Autodesk Inventor part; units mm, degrees
ref_plane "YZ Plane" through (0, 0, 0) normal (1, 0, 0) x (0, 1, 0)
ref_plane "XZ Plane" through (0, 0, 0) normal (0, 1, 0) x (-1, 0, 0)
ref_plane "XY Plane" through (0, 0, 0) normal (0, 0, 1) x (1, 0, 0)
sketch "Sketch1" plane through (0, 0, 0) normal (0, 0, 1) x (1, 0, 0)
  line L0 (0, 0) -> (76, 0)
  line L1 (76, 0) -> (76, -8)
  line L2 (76, -8) -> (0, -8)
  line L3 (0, -8) -> (0, 0)
  dimension "d0" = 76
  dimension "d1" = 8
extrude "Extrusion1" add sketch "Sketch1" along normal blind 3
sketch "Sketch2" plane through (0, 0, 3) normal (0, 0, 1) x (1, 0, 0)
  line L0 (0, 0) -> (0, -8)
  circle A0 centre (0, -4) radius 1.9
  line L1 (76, -8) -> (76, 0)
  circle A1 centre (76, -4) radius 1.9
  dimension "d4" = 3.8
  dimension "d5" = 3.8
extrude "Extrusion2" add sketch "Sketch2" along normal blind 6
sketch "Sketch3" plane through (0, 0, 0) normal (0, 0, -1) x (-1, 0, 0)
  line L0 (0, -8) -> (-76, -8)
  line L1 (0, -8) -> (2.5, -8)
  line L2 (2.5, -8) -> (2.5, 0)
  line L3 (2.5, 0) -> (0, 0)
  line L4 (0, 0) -> (0, -8)
  line L5 (-76, -8) -> (-78.5, -8)
  line L6 (-78.5, -8) -> (-78.5, 0)
  line L7 (-78.5, 0) -> (-76, 0)
  line L8 (-76, 0) -> (-76, -8)
  dimension "d8" = 2.5
  dimension "d9" = 2.5
extrude "Extrusion3" add sketch "Sketch3" against normal blind 3
properties part number "SteeringWheel"
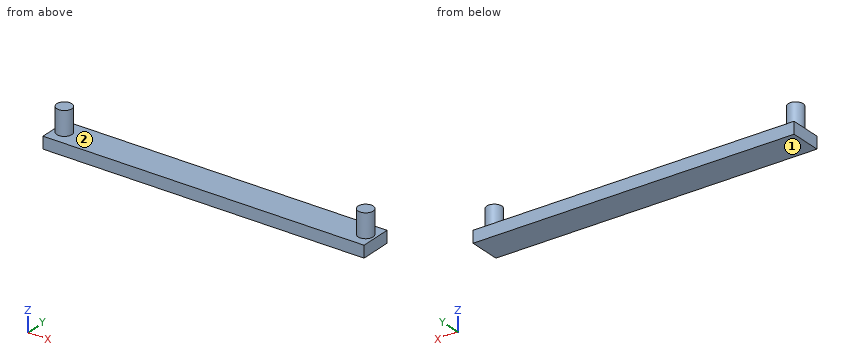
Source: CAD feature listing. Evaluate the final solid. Frame: model axes, mm. Face numbers are marked on the shaded views. Coordinates: 2 decimals unless noted, no trailing zeros. Write each loop counter-clockwise with the first axis right and the second up, starting at its lowest first coordinate (ties: lowest second). Pieces come first, ordered by that corner, then holes. Notation, with made-up numbers: M 60,-24.5 L 107,-24.5 A19 ccw 107,-6.5 Z; hole C 69,67 d6. An arc over 180 degrees is marked long. Use a Markdown table: item, result.
1) Section D-D, the plane x = 25.5. Output: boundary loops of the cut face in (y, z).
Conclusion:
| item | result |
|---|---|
| outline | M -8,0 L 0,0 L 0,3 L -8,3 Z |
2) Section B-B, the plane y = -4. Output: boundary loops of the cut face in (x, z).
Conclusion:
| item | result |
|---|---|
| outline | M -2.5,0 L 78.5,0 L 78.5,3 L 77.9,3 L 77.9,9 L 74.1,9 L 74.1,3 L 1.9,3 L 1.9,9 L -1.9,9 L -1.9,3 L -2.5,3 Z |
3) First-contact query: pin 1 Ø1.5 at (x, z) = (55, 2) entering from +Y; pin 2 Ø4 at (x, y) = (42, -2) entering from +Z. Flat tips, straight axial feed; report the tip coordinate or a pass-through.
Conclusion:
| item | result |
|---|---|
| pin 1 | stops at y = 0 |
| pin 2 | stops at z = 3 |
4) Ray query, L1, parallel to Z at x = 60.5, y = -4.75; L2, parallel to X at y = -4, z = 8; L3, parallel to X at y = -2.75, z = 6. Return the intervals inside material, ascending.
Conclusion:
| item | result |
|---|---|
| L1 | z = 0 to 3 |
| L2 | x = -1.9 to 1.9, 74.1 to 77.9 |
| L3 | x = -1.43 to 1.43, 74.57 to 77.43 |
5) Section A-A, the plane x = 0. Output: boundary loops of the cut face in (y, z), then the cut area to 3 significant figures.
Conclusion:
| item | result |
|---|---|
| outline | M -8,0 L 0,0 L 0,3 L -2.1,3 L -2.1,9 L -5.9,9 L -5.9,3 L -8,3 Z |
| area | 46.8 mm^2 |
6) Mould query, pull axis X, two halves, no side actions, for the marked faces 1 and 2. Classes: pulls with the +X half, pulls with the -X half, needs draft (parallel to the pull), parting line crosses it, or undercut.
Conclusion:
| item | result |
|---|---|
| face 1 | needs draft |
| face 2 | undercut |
7) Section C-C, the plane z = 7.25. Output: boundary loops of the cut face in (x, y), then the cut area to 3 significant figures.
Conclusion:
| item | result |
|---|---|
| outline | C 0,-4 d3.8; C 76,-4 d3.8 |
| area | 22.7 mm^2 |
